from build123d import *

# Parameters (mm, degrees)
SKETCH_1_W          = 106
SKETCH_1_H          = 106
SKETCH_1_R          = 1.5
SKETCH_1_W_2        = 72
SKETCH_1_H_2        = 25
SKETCH_1_W_3        = 90
SKETCH_1_H_3        = 56
EXTRUDE_1_DEPTH     = 10
SKETCH_2_W          = 106
SKETCH_2_H          = 106
SKETCH_2_W_2        = 102
SKETCH_2_H_2        = 102
CUT_EXTRUDE_1_DEPTH = 4
SKETCH_3_W          = 81
SKETCH_3_H          = 36.6
CUT_EXTRUDE_2_DEPTH = 6
SKETCH_4_W          = 89.344385993
SKETCH_4_H          = 1.858759764
CUT_EXTRUDE_3_DEPTH = 7
CUT_EXTRUDE_4_DEPTH = 4
CUT_EXTRUDE_5_DEPTH = 3
SKETCH_8_W          = 26
SKETCH_8_H          = 17.490205858
CUT_EXTRUDE_6_DEPTH = 2


with BuildPart() as part:
    # 草图1 → 凸台-拉伸1 (new body)
    with BuildSketch(Plane.XY):
        with Locations((53, 53)):
            Rectangle(SKETCH_1_W, SKETCH_1_H)
        with Locations((3.324461644, 102.636394846)):
            Circle(SKETCH_1_R, mode=Mode.SUBTRACT)
        with Locations(Location((102.675538356, 102.636394846, 0), (0, 0, 180))):
            Circle(SKETCH_1_R, mode=Mode.SUBTRACT)
        with Locations((102.675538356, 3.363605154)):
            Circle(SKETCH_1_R, mode=Mode.SUBTRACT)
        with Locations(Location((3.324461644, 3.363605154, 0), (0, 0, 180))):
            Circle(SKETCH_1_R, mode=Mode.SUBTRACT)
        with Locations((53, 84.537117037)):
            Rectangle(SKETCH_1_W_2, SKETCH_1_H_2, mode=Mode.SUBTRACT)
        with Locations((53, 35.575547917)):
            Rectangle(SKETCH_1_W_3, SKETCH_1_H_3, mode=Mode.SUBTRACT)
    extrude(amount=EXTRUDE_1_DEPTH)

    # 草图2 → 切除-拉伸1 (cut)
    with BuildSketch(Plane.XY.offset(10)):
        with Locations((53, 53)):
            Rectangle(SKETCH_2_W, SKETCH_2_H)
        with Locations((53, 53)):
            Rectangle(SKETCH_2_W_2, SKETCH_2_H_2, mode=Mode.SUBTRACT)
    extrude(amount=-CUT_EXTRUDE_1_DEPTH, mode=Mode.SUBTRACT)

    # 草图3 → 切除-拉伸2 (cut)
    with BuildSketch(Plane.XY.offset(10)):
        with Locations((53, 84.537117037)):
            Rectangle(SKETCH_3_W, SKETCH_3_H)
    extrude(amount=-CUT_EXTRUDE_2_DEPTH, mode=Mode.SUBTRACT)

    # 草图4 → 切除-拉伸3 (cut)
    with BuildSketch(Plane.XY.offset(10)):
        Polygon((4.238535523, 99.03528349), (5.849460651, 99.03528349), (5.849460651, 101.885381795), (10.06264945, 101.885381795), (10.06264945, 66.237117037), (5.849460651, 66.237117037), (5.849460651, 7.708220416), (4.238535523, 7.708220416), align=None)
        Polygon((95.93735055, 66.237117037), (100.150539349, 66.237117037), (100.150539349, 7.708220416), (101.761464477, 7.708220416), (101.761464477, 99.03528349), (100.150539349, 99.03528349), (100.150539349, 101.885381795), (95.93735055, 101.885381795), align=None)
        with Locations((52.752165365, 4.920080769)):
            Rectangle(SKETCH_4_W, SKETCH_4_H)
    extrude(amount=-CUT_EXTRUDE_3_DEPTH, mode=Mode.SUBTRACT)

    # 草图5 → 切除-拉伸4 (cut)
    with BuildSketch(Plane.XY.offset(10)):
        Polygon((7.956055051, 101.885381795), (98.043944949, 101.885381795), (98.043944949, 66.237117037), (100.150539349, 66.237117037), (100.150539349, 5.849460651), (5.849460651, 5.849460651), (5.849460651, 66.237117037), (7.956055051, 66.237117037), align=None)
    extrude(amount=-CUT_EXTRUDE_4_DEPTH, mode=Mode.SUBTRACT)

    # 草图6 → 切除-拉伸5 (cut)
    with BuildSketch(Plane.XY.offset(4)):
        Polygon((17, 97.037117037), (12.5, 91.104575163), (12.5, 78.34109145), (17, 72.037117037), align=None)
        Polygon((89, 72.037117037), (89, 97.037117037), (93.5, 91.104575163), (93.5, 78.34109145), align=None)
    extrude(amount=-CUT_EXTRUDE_5_DEPTH, mode=Mode.SUBTRACT)

    # 草图8 → 切除-拉伸6 (cut)
    with BuildSketch(Plane.XY.offset(10)):
        with Locations((53, 3.253738618)):
            Rectangle(SKETCH_8_W, SKETCH_8_H)
    extrude(amount=-CUT_EXTRUDE_6_DEPTH, mode=Mode.SUBTRACT)


solid = part.part
Part model, mm, in its own coordinate system. A direction names the side the tool comes from. Round coordinates to 2 decimals unless told otherwise and drop trailing zeros. Order: outer loops, then holes, each group sorted by start corner. A loop starts at its lowest first (then second) coordinate and runs counter-clockwise, first axis right, second up. Notation, with made-up numbers: (49, 17.25) -> (65, 17.25) arc R21 cw to (65, 50.25) -> close; hole circle Ø4 at (8.5, 0.25). An arc over 180 degrees is marked (long way). Put each result on its own line as item: value.
Q1. Band-saw the part on C-C (y = 80.5). Give the cut face in (x, z).
From the geometry:
outline: (0, 0) -> (17, 0) -> (17, 1) -> (12.5, 1) -> (12.5, 6) -> (10.06, 6) -> (10.06, 3) -> (4.24, 3) -> (4.24, 10) -> (2, 10) -> (2, 6) -> (0, 6) -> close; (89, 0) -> (106, 0) -> (106, 6) -> (104, 6) -> (104, 10) -> (101.76, 10) -> (101.76, 3) -> (95.94, 3) -> (95.94, 6) -> (93.5, 6) -> (93.5, 1) -> (89, 1) -> close
Q2. Pull direction X, two halves, no side cores. Call faces 1 (the face through (91, 85, 1)), 2 (the face through (0, 52, 3)), 3 (the face through (52.3, 2, 7.6)): pulls with the +X half, pulls with the -X half, needs draft (parallel to the pull), parting line crosses it, or undercut.
From the geometry:
face 1: undercut
face 2: pulls with the -X half
face 3: needs draft
Q3. Tool access for faces 4 (the face through (12.5, 86, 5)), 5 (the face through (52, 106, 3)), 6 (the face through (98, 35, 3)): list every direction of +Z, -Z, +X, -X, +Y, -Y with a clear straight run to the whole face (end or side of a thin tool).
From the geometry:
face 4: +Z
face 5: +Z, -Z, +X, -X, +Y
face 6: +Z, -Z
Q4. Wall check: line 1 (Y direction, x = 28, z = 2.5); line 2 (Y direction, x = 38, z = 3.5); line 3 (Y direction, x = 71, z = 4.75). Give the ranges that are in metal, low to high. Write a range as [from, to].
From the geometry:
line 1: y = [0, 7.58], [63.58, 72.04], [97.04, 106]
line 2: y = [0, 3.99], [5.85, 7.58], [63.58, 72.04], [97.04, 106]
line 3: y = [0, 3.99], [5.85, 7.58], [63.58, 66.24], [102.84, 106]
Q5. Band-saw the part on A-A (x = 47.5). Give the cut face in (y, z).
From the geometry:
outline: (0, 0) -> (7.58, 0) -> (7.58, 6) -> (5.85, 6) -> (5.85, 3) -> (3.99, 3) -> (3.99, 8) -> (2, 8) -> (2, 6) -> (0, 6) -> close; (63.58, 0) -> (72.04, 0) -> (72.04, 4) -> (66.24, 4) -> (66.24, 6) -> (63.58, 6) -> close; (97.04, 0) -> (106, 0) -> (106, 6) -> (104, 6) -> (104, 10) -> (102.84, 10) -> (102.84, 4) -> (97.04, 4) -> close
Q6. Band-saw the part on B-B (y = 41.5). Give the cut face in (x, z), and give its area (3 significant figures).
From the geometry:
outline: (0, 0) -> (8, 0) -> (8, 6) -> (5.85, 6) -> (5.85, 3) -> (4.24, 3) -> (4.24, 10) -> (2, 10) -> (2, 6) -> (0, 6) -> close; (98, 0) -> (106, 0) -> (106, 6) -> (104, 6) -> (104, 10) -> (101.76, 10) -> (101.76, 3) -> (100.15, 3) -> (100.15, 6) -> (98, 6) -> close
area: 104 mm2
Q7. Pin check, flat tips, straight feed: pin 1 Ø1.5 at (y, z) = (7, 9) entering from +X; pin 2 Ø6 at (x, z) = (72, 5.5) entering from -Y; pin 3 Ø5 at (x, y) = (16, 81.5) entering from +Z; pin 4 Ø9.5 at (x, y) = (50.5, 72) entering from +Z. Stop position of each tip, or through.
From the geometry:
pin 1: stops at x = 104
pin 2: stops at y = 0
pin 3: stops at z = 1
pin 4: stops at z = 4
